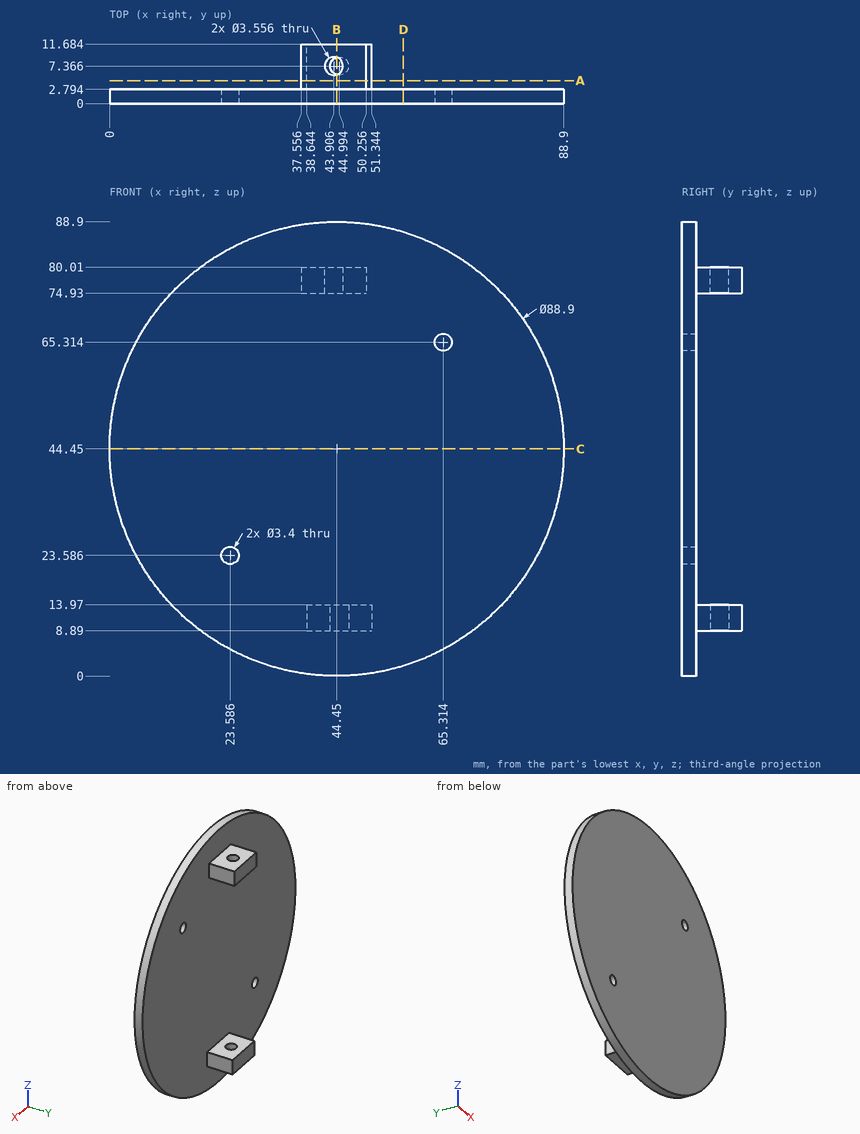
Could you check a few things on this drawing? It's one solid part, dimensions in mm from its lowest x, y, z. Round coordinates to 2 decimals unless told otherwise and drop trailing zeros. Order: outer loops, then holes, each group sorted by start corner. A loop starts at its lowest first (then second) coordinate and runs counter-clockwise, first axis right, second up.
Q1. Imagine slicing it at A-A, the plane y = 4.5. List the corners of the cut face in (x, z) for me, then the cut area to 3 significant figures.
Geometry says:
outline: (37.56, 74.93) - (50.26, 74.93) - (50.26, 80.01) - (37.56, 80.01) - close; (38.64, 8.89) - (51.34, 8.89) - (51.34, 13.97) - (38.64, 13.97) - close
area: 129 mm2
Q2. I'm going to push flat-ended pins straight in: P1, Ø4, axis at y = 7, z = 12, coming from the +X side; P2, Ø4, axis at y = 6, z = 78, coming from the -X side; P3, Ø6, axis at x = 39, y = 9.5, coming from the +Z side. Where does each tip first touch, or does it pass through?
Geometry says:
P1: stops at x = 51.34
P2: stops at x = 37.56
P3: stops at z = 80.01
Q3. Imagine slicing it at D-D, the plane x = 57.5. List the corners of the cut face in (y, z) for me, then the cut area to 3 significant figures.
Geometry says:
outline: (0, 1.96) - (2.79, 1.96) - (2.79, 86.94) - (0, 86.94) - close
area: 237 mm2
Q4. Imagine slicing it at C-C, the plane z = 44.45. List the corners of the cut face in (x, y) for me, then the cut area to 3 significant figures.
Geometry says:
outline: (0, 0) - (88.9, 0) - (88.9, 2.79) - (0, 2.79) - close
area: 248 mm2
Q5. Please list where these lines run through material, in increasing order: probe 1 along Z at (x, y) = (43, 10); probe 2 along Y at (x, z) = (43, 34); probe 3 along X at (y, z) = (2.5, 13).
Geometry says:
probe 1: z = 8.89 to 13.97, 74.93 to 80.01
probe 2: y = 0 to 2.79
probe 3: x = 13.04 to 75.86
Q6. Imagine slicing it at B-B, the plane x = 44.45. List the corners of the cut face in (y, z) for me.
Geometry says:
outline: (0, 0) - (2.79, 0) - (2.79, 8.89) - (5.67, 8.89) - (5.67, 13.97) - (2.79, 13.97) - (2.79, 74.93) - (5.67, 74.93) - (5.67, 80.01) - (2.79, 80.01) - (2.79, 88.9) - (0, 88.9) - close; (9.06, 8.89) - (11.68, 8.89) - (11.68, 13.97) - (9.06, 13.97) - close; (9.06, 74.93) - (11.68, 74.93) - (11.68, 80.01) - (9.06, 80.01) - close
